Build history of the part. All positions in model axes, mm. Round coordinates to 2 decimals unless told otherwise and drop trailing zeros. Write each loop counter-clockwise with the first axis right and the second up, starting at its lowest first coordinate (ties: lowest second). Pieces come first, ordered by that corner, then holes. Notation, with made-up numbers: M -9.5,-8.75 L 38.5,-8.75 A20 ccw 38.5,14.25 Z; hole C -17,-16.75 d2. An arc over 180 degrees is marked long. Use a Markdown table: item, result.
from build123d import *

# Parameters (mm, degrees)
F0_W     = 10
F0_H     = 10
F1_DEPTH = 7
F2_DEPTH = 1
F3_W     = 18
F3_H     = 6
F4_DEPTH = 504


with BuildPart() as f1:
    # F0 (on Top) → F1 (new body)
    with BuildSketch(Plane.XY):
        Polygon((336.860095, -249.837965), (-168.139905, -249.837965), (-168.139905, -254.837965), (-158.139905, -254.837965), (-158.139905, -264.837965), (-168.139905, -264.837965), (-168.139905, -269.837965), (336.860095, -269.837965), align=None)
        with Locations((-163.139905, -259.837965)):
            Rectangle(F0_W, F0_H)
    extrude(amount=F1_DEPTH)

    # F0 (on Top) → F2 (join)
    with BuildSketch(Plane.XY):
        with Locations((-163.139905, -259.837965)):
            Rectangle(F0_W, F0_H)
    extrude(amount=-F2_DEPTH)

    # F3 (on face) → F4 (cut)
    with BuildSketch(Plane(origin=(-168.139905, 0, 0), x_dir=(0, -1, 0), z_dir=(-1, 0, 0))):
        with Locations((259.837965, 3.5)):
            Rectangle(F3_W, F3_H)
    extrude(amount=-F4_DEPTH, mode=Mode.SUBTRACT)


solid = f1.part
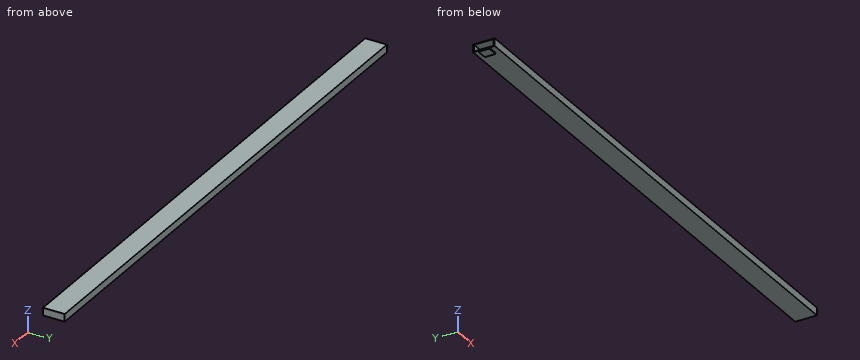
Q1. Drop flat-ended pins along their axis: P1, Ø5, axis at x = -46.5, y = -253, coming from the -Z side; P2, Ø0.8, axis at y = -259, z = -0.5, coming from the +X side; P3, Ø3, axis at y = -256.5, z = 2.5, coming from the -X side. Give the stop position or say it passes through.
Response values:
| item | result |
|---|---|
| P1 | stops at z = 0 |
| P2 | stops at x = -158.14 |
| P3 | stops at x = 335.86 |
Q2. Drill centre lines: L1, parallel to Y at x = 13.5, z = 1.5; L2, parallel to Z at x = 65, y = -257.25; L3, parallel to X at y = -261.25, z = 5. Where is each one in solid material? Low to high.
Response values:
| item | result |
|---|---|
| L1 | y = -269.84 to -268.84, -250.84 to -249.84 |
| L2 | z = 0 to 0.5, 6.5 to 7 |
| L3 | x = 335.86 to 336.86 |
Q3. Cut at B-B on z = 4. Give the cut face in (x, y), and give its area (3 significant figures).
Response values:
| item | result |
|---|---|
| outline | M -168.14,-269.84 L 336.86,-269.84 L 336.86,-249.84 L -168.14,-249.84 L -168.14,-250.84 L 335.86,-250.84 L 335.86,-268.84 L -168.14,-268.84 Z |
| area | 1,030 mm2 |
Q4. Cut at A-A on x = 273. Give the cut face in (y, z), and give its area (3 significant figures).
Response values:
| item | result |
|---|---|
| outline | M -269.84,0 L -249.84,0 L -249.84,7 L -269.84,7 Z; hole M -268.84,0.5 L -250.84,0.5 L -250.84,6.5 L -268.84,6.5 Z |
| area | 32.0 mm2 |
Q5. Cut at C-C on y = -260.75. Give the cut face in (x, z).
Response values:
| item | result |
|---|---|
| outline | M -168.14,-1 L -158.14,-1 L -158.14,0 L 336.86,0 L 336.86,7 L -168.14,7 L -168.14,6.5 L 335.86,6.5 L 335.86,0.5 L -168.14,0.5 Z |
